Drawing for the job (mm, zero at the part's lowest x, y, z). Give positions to 0.01 mm unless a question says otherwise; leave off trailing zeros. Write each loop counter-clockwise with the first axis right and the second up, starting at its lowest first coordinate (ties: lowest second). Pieces come first, ordered by that corner, then holes.
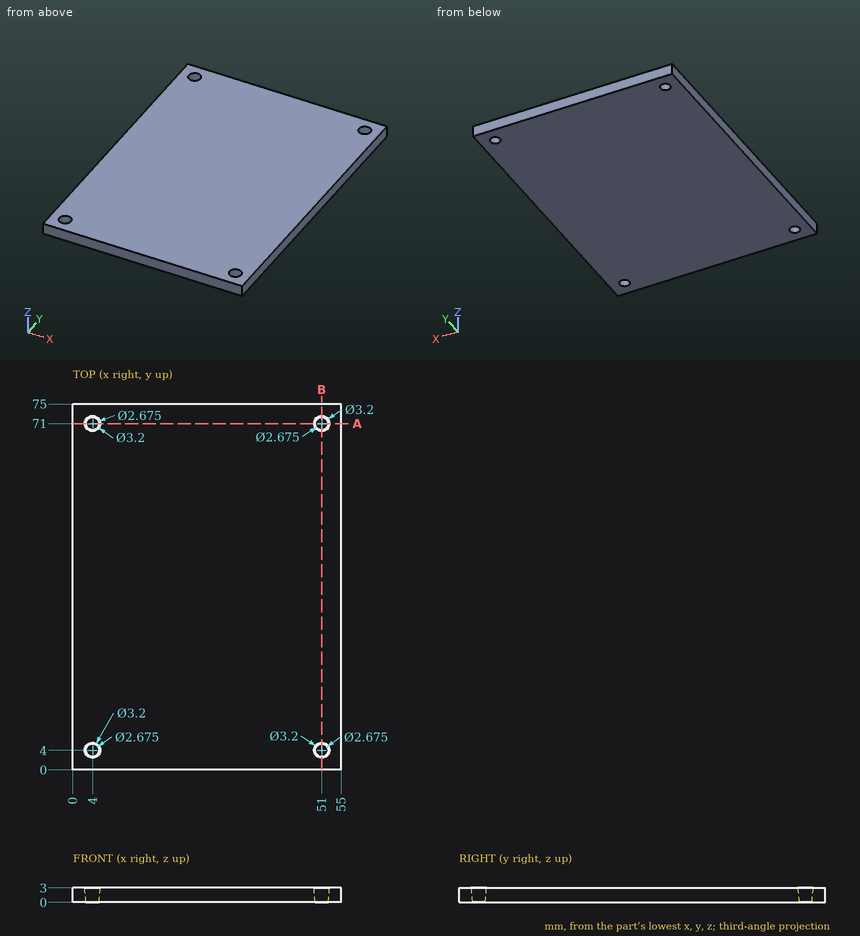
1. Slice it at B-B, the plane x = 51. Write the cut outline in (y, z), and give its area (3 significant figures).
Calculated:
outline: (0, 0) - (2.66, 0) - (2.4, 3) - (0, 3) - close; (5.34, 0) - (69.66, 0) - (69.4, 3) - (5.6, 3) - close; (72.34, 0) - (75, 0) - (75, 3) - (72.6, 3) - close
area: 207 mm2
2. Slice it at A-A, the plane y = 71. Write the cut outline in (x, z), and give its area (3 significant figures).
Calculated:
outline: (0, 0) - (2.66, 0) - (2.4, 3) - (0, 3) - close; (5.34, 0) - (49.66, 0) - (49.4, 3) - (5.6, 3) - close; (52.34, 0) - (55, 0) - (55, 3) - (52.6, 3) - close
area: 147 mm2
3. Probe probe 1 along X at (y, z) = (4, 1.45). List the from-to ranges inside material, lowest first.
Calculated:
probe 1: x = 0 to 2.54, 5.46 to 49.54, 52.46 to 55
4. Pin check, flat tip, straight feed: P1, Ø1.5, axis at x = 18.5, z = 1, coming from the -Y side. Stop position of the tip, or through.
Calculated:
P1: stops at y = 0
